from build123d import *

# Parameters (mm, degrees)
BOSS_EXTRUDE1_DEPTH     = 2
BOSS_EXTRUDE2_DEPTH     = 10
CUT_EXTRUDE1_DEPTH      = 119.595420067
CUT_EXTRUDE1_DEPTH_BACK = 119.595420067


with BuildPart() as part:
    # Sketch1 → Boss-Extrude1 (new body)
    with BuildSketch(Plane.XY):
        with BuildLine():
            Line((-48.55615004, 95.168805411), (29.960861776, 95.168805411))
            ThreePointArc((29.960861776, 95.168805411), (44.1029974, 89.310941035), (49.960861776, 75.168805411))
            Line((49.960861776, 75.168805411), (49.960861776, -76.254495753))
            ThreePointArc((49.960861776, -76.254495753), (44.1029974, -90.396631376), (29.960861776, -96.254495753))
            Line((29.960861776, -96.254495753), (-48.556149966, -96.254495753))
            ThreePointArc((-48.556149966, -96.254495753), (-62.698285587, -90.39663138), (-68.556149966, -76.254495762))
            Line((-68.556149966, -76.254495762), (-68.55615004, 75.168805401))
            ThreePointArc((-68.55615004, 75.168805401), (-62.698285667, 89.310941031), (-48.55615004, 95.168805411))
        make_face()
    extrude(amount=BOSS_EXTRUDE1_DEPTH)

    # Sketch1_3 → Boss-Extrude2 (add)
    with BuildSketch(Plane.XY):
        with BuildLine():
            Line((-48.55615004, 85.168805411), (29.960861776, 85.168805411))
            ThreePointArc((29.960861776, 85.168805411), (37.031929588, 82.239873223), (39.960861776, 75.168805411))
            Line((39.960861776, 75.168805411), (39.960861776, -44.933857001))
            ThreePointArc((39.960861776, -44.933857001), (37.031929588, -52.004924813), (29.960861776, -54.933857001))
            Line((29.960861776, -54.933857001), (-48.556149982, -54.933857001))
            ThreePointArc((-48.556149982, -54.933857001), (-55.627217792, -52.004924815), (-58.556149982, -44.933857006))
            Line((-58.556149982, -44.933857006), (-58.55615004, 75.168805406))
            ThreePointArc((-58.55615004, 75.168805406), (-55.627217853, 82.239873221), (-48.55615004, 85.168805411))
        make_face()
        with BuildLine():
            Line((-48.55615004, 83.168805411), (29.960861776, 83.168805411))
            ThreePointArc((29.960861776, 83.168805411), (35.617716026, 80.82565966), (37.960861776, 75.168805411))
            Line((37.960861776, 75.168805411), (37.960861776, -44.933856987))
            ThreePointArc((37.960861776, -44.933856987), (35.617716026, -50.590711236), (29.960861776, -52.933856987))
            Line((29.960861776, -52.933856987), (-48.556149982, -52.933856987))
            ThreePointArc((-48.556149982, -52.933856987), (-54.21300423, -50.590711237), (-56.556149982, -44.93385699))
            Line((-56.556149982, -44.93385699), (-56.55615004, 75.168805407))
            ThreePointArc((-56.55615004, 75.168805407), (-54.213004291, 80.825659659), (-48.55615004, 83.168805411))
        make_face(mode=Mode.SUBTRACT)
    extrude(amount=-BOSS_EXTRUDE2_DEPTH)

    # Sketch3 → Cut-Extrude1 (cut, two sides: drawn at the far end of the back side and taken through both)
    with BuildSketch(Plane(origin=(0, 0, 0), x_dir=(-1, 0, 0), z_dir=(0, 0, -1)).offset(-CUT_EXTRUDE1_DEPTH_BACK)):
        with BuildLine():
            Line((25.489402973, -36.700798798), (25.595818918, -10.417445008))
            add(Edge.make_bspline(
                [(25.595818918, -10.417445008), (25.595818918, -1.296173206), (12.173879387, -1.295746312), (-1.248060145, -1.295319417), (-1.249316495, -10.416591179)],
                knots=[0, 0, 0, 1.570749525, 1.570749525, 3.141499049, 3.141499049, 3.141499049], degree=2, weights=[1, 0.707123328, 1, 0.707123328, 1]))
            Line((-1.249316495, -10.416591179), (-1.253050558, -37.527526675))
            add(Edge.make_bspline(
                [(-1.253050558, -37.527526675), (0.598808841, -42.641507472), (13.044105907, -42.256768128), (25.489402973, -41.872028784), (25.489402973, -36.700798798)],
                knots=[0.148937555, 0.148937555, 0.148937555, 1.645265104, 1.645265104, 3.141592654, 3.141592654, 3.141592654], degree=2, weights=[1, 0.732939277, 1, 0.732939277, 1]))
        make_face()
    extrude(amount=CUT_EXTRUDE1_DEPTH + CUT_EXTRUDE1_DEPTH_BACK, mode=Mode.SUBTRACT)


solid = part.part
Here's how the part is built. I have some questions about the finished solid (model axes, mm). A direction names the side the tool comes from. Coordinates: 2 decimals unless noted, no trailing zeros. Write each loop counter-clockwise with the first axis right and the second up, starting at its lowest first coordinate (ties: lowest second). Pieces come first, ordered by that corner, then holes.
1) If we section it at D-D (y = -15): List the corners of the cut face in (x, z) for me.
Filled in:
outline: (-68.56, 0) - (-58.56, 0) - (-58.56, -10) - (-56.56, -10) - (-56.56, 0) - (-25.58, 0) - (-25.58, 2) - (-68.56, 2) - close; (1.25, 0) - (37.96, 0) - (37.96, -10) - (39.96, -10) - (39.96, 0) - (49.96, 0) - (49.96, 2) - (1.25, 2) - close
2) Which directions (+Z, -Z, +X, -X, +Y, -Y) give clear straight access to the entire face, cutting with the end or side of a thin tool? Please do faces 5 (the face through (36.95, 82.32, -4.93)), 6 (the face through (-55.55, -52.08, -4.93)), 7 (the face through (-56.556, 14, -5)), 8 (the face through (-55.705, 82.162, -4.93)).
Filled in:
face 5: -Z, +X, +Y
face 6: -Z, -X, -Y
face 7: -Z
face 8: -Z, -X, +Y
3) If we section it at C-C (x = 16.5): List the corners of the cut face in (y, z) for me.
Filled in:
outline: (-96.25, 0) - (-54.93, 0) - (-54.93, -10) - (-52.93, -10) - (-52.93, 0) - (83.17, 0) - (83.17, -10) - (85.17, -10) - (85.17, 0) - (95.17, 0) - (95.17, 2) - (-96.25, 2) - close
4) I'm going to push flat-ended pins straight in: pin 1 (1 mm diameter, centred on x = 35, z = -3, fed in from -Y); pin 2 (1.5 mm diameter, centred on x = 30, z = -3, fed in from +Y); pin 3 (3 mm diameter, centred on y = 35.5, z = -4.5, fed in from +X). Where does each tip first touch, or does it pass through?
Filled in:
pin 1: stops at y = -53.84
pin 2: stops at y = 85.17
pin 3: stops at x = 39.96
5) Thinking about a two-plate mould opening in Y: for faces 1 (the face through (37.109, -51.927, -4.93)), 2 (the face through (-10, 83.169, -5)), 3 (the face through (-8, -63, 0)), 4 (the face through (-54.275, 80.763, -4.93)), which applies, +Y half, -Y half, draft (parallel to the pull), parting line (faces both ways), or undercut?
Filled in:
face 1: -Y half
face 2: undercut
face 3: draft
face 4: undercut
6) If I drill on line 1 (X direction, y = 3.5, z = -6.5); line 2 (Y direction, x = 28, z = -7); line 3 (Z direction, x = 22.5, y = -34), over which ranges is the centre line in solid material (lowest first)?
Filled in:
line 1: x = -58.56 to -56.56, 37.96 to 39.96
line 2: y = -54.93 to -52.93, 83.17 to 85.17
line 3: z = 0 to 2
7) If we section it at A-A (z = -4.5): List the corners of the cut face in (x, y) for me, plus the area to 3 significant figures.
Filled in:
outline: (-58.56, -44.93) arc R10 ccw to (-48.56, -54.93) - (29.96, -54.93) arc R10 ccw to (39.96, -44.93) - (39.96, 75.17) arc R10 ccw to (29.96, 85.17) - (-48.56, 85.17) arc R10 ccw to (-58.56, 75.17) - close; hole (-56.56, -44.93) arc R8 ccw to (-48.56, -52.93) - (29.96, -52.93) arc R8 ccw to (37.96, -44.93) - (37.96, 75.17) arc R8 ccw to (29.96, 83.17) - (-48.56, 83.17) arc R8 ccw to (-56.56, 75.17) - close
area: 908 mm2
8) If we section it at B-B (y = 37): List the corners of the cut face in (x, z) for me, plus the area to 3 significant figures.
Filled in:
outline: (-68.56, 0) - (-58.56, 0) - (-58.56, -10) - (-56.56, -10) - (-56.56, 0) - (37.96, 0) - (37.96, -10) - (39.96, -10) - (39.96, 0) - (49.96, 0) - (49.96, 2) - (-68.56, 2) - close
area: 277 mm2
